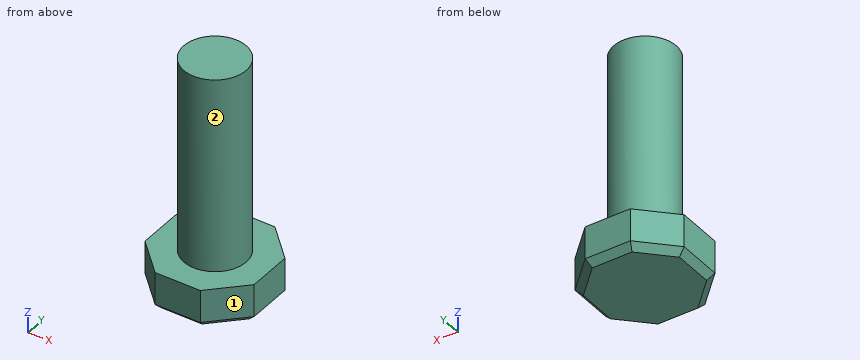
from build123d import *

# Parameters (mm, degrees)
EXTRUDE2_DEPTH = 15
CHAMFER3_SIZE  = 2.5
SKETCH3_R      = 12
EXTRUDE3_DEPTH = 75


with BuildPart() as part:
    # Sketch2 → Extrude2 (new body)
    with BuildSketch(Plane.XY):
        Polygon((-21, 8.69848481), (-8.69848481, 21), (8.69848481, 21), (21, 8.69848481), (21, -8.69848481), (8.69848481, -21), (-8.69848481, -21), (-21, -8.69848481), align=None)
    extrude(amount=EXTRUDE2_DEPTH)

    # Chamfer3
    chamfer3_edges = [part.edges().sort_by_distance(p)[0] for p in [
        (14.849242405, 14.849242405, 0),
        (21, 0, 0),
        (14.849242405, -14.849242405, 0),
        (0, -21, 0),
        (-14.849242405, -14.849242405, 0),
        (-21, 0, 0),
        (-14.849242405, 14.849242405, 0),
        (0, 21, 0),
    ]]
    chamfer(chamfer3_edges, length=CHAMFER3_SIZE)

    # Sketch3 → Extrude3 (add)
    with BuildSketch(Plane.XY.offset(15)):
        with Locations(Location((0, 0, 0), (0, 0, 180))):
            Circle(SKETCH3_R)
    extrude(amount=EXTRUDE3_DEPTH)


solid = part.part
Check sheet for the modelled part. Datum: model origin and axes. Units: mm. Face numbers are marked on the shaded views. A direction names the side the tool comes from. Coordinates: 2 decimals unless noted, no trailing zeros. Write each loop counter-clockwise with the first axis right and the second up, starting at its lowest first coordinate (ties: lowest second). Pieces come first, ordered by that corner, then holes. Notation, with made-up numbers: M 56,12 L 106,12 A28 ccw 106,38 Z; hole C 55.5,37 d3. An arc over 180 degrees is marked long. Answer as CSV lines item,"result".
Q1. Go/stop test with flat-tipped pins: pin 1 (4 mm diameter, centred on x = -8.5, z = 26, fed in from -Y); pin 2 (8 mm diameter, centred on x = 13, z = 68.5, fed in from +Y); pin 3 (6 mm diameter, centred on x = -6, z = 79.5, fed in from -Y). Record where each tip stops, or that it passes through.
Check result:
pin 1,"y = -10.09"
pin 2,"y = 7.94"
pin 3,"y = -11.62"
Q2. Cross-section at A-A (x = 0). Record the boundary of the cut face in (y, z).
Check result:
outline,"M -21,2.5 L -18.5,0 L 18.5,0 L 21,2.5 L 21,15 L 12,15 L 12,90 L -12,90 L -12,15 L -21,15 Z"
Q3. Material ranges on probe 1 along Z at (x, y) = (12, 11.5); probe 2 along Y at (x, z) = (-15.5, 14.5); probe 3 along Y at (x, z) = (4, 85.5), recorded low to high. Write a range as from..to.
Check result:
probe 1,"0..15"
probe 2,"-14.2..14.2"
probe 3,"-11.31..11.31"
Q4. Cross-section at C-C (z = 65). Record the boundary of the cut face in (x, y), then the cut area to 3 significant figures.
Check result:
outline,"C 0,0 d24"
area,"452 mm^2"
Q5. Set-up check for the marked faces 1 and 2: record each of +Z, -Z, +X, -X, +Y, -Y from which the full face is reachable in a straight line by a thin tool's end or side.
Check result:
face 1,"+Z, -Z, +X, -Y"
face 2,"+Z"
